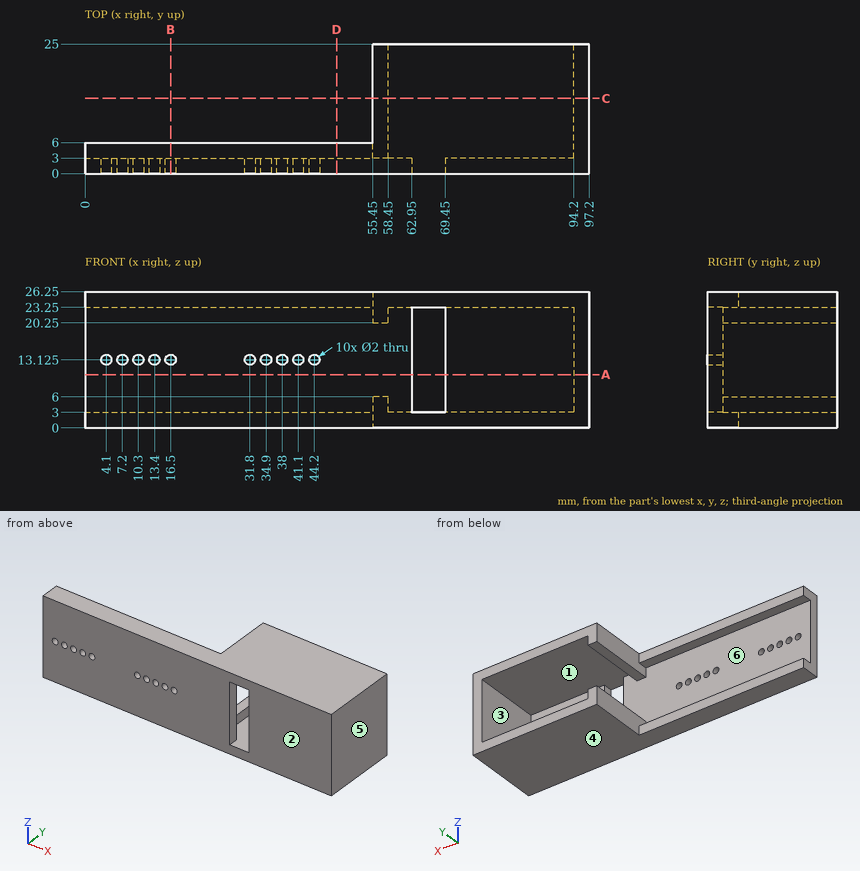
Input: dimensioned drawing with shaded views. Units: mm. Origin: part minimum x, y, z. A direction names the side the tool comes from. Give positions to 0.01 mm unless a question says otherwise; leave off trailing zeros. Order: outer loops, then holes, each group sorted by start corner. A loop starts at its lowest first (then second) coordinate and runs counter-clockwise, first axis right, second up.
(1) Access query for the marked faces 1 and 2. Directions: +Z, -Z, +X, -X, +Y, -Y. A direction counts if a zero-diameter tool reaches every point of the face in a straight line with its end or side. Return the directions, or none.
(2) Contact query for flat-ended pins moving along their axis: P1, Ø1, axis at x = 14, z = 18, coming from the +Y side; P2, Ø3, axis at y = 19.5, z = 22.5, coming from the -X side; P3, Ø0.9, axis at x = 26, z = 24.5, coming from the +Y side. Output: stop coordinate, or through.
(3) Pull-direction query (Z, two-part tool) for the marked faces 3, 4, 5 and 6; classes: +Z half, -Z half, draft (parallel to the pull), parting line (faces both ways), or undercut.
(4) Section query C-C (y = 14.5). Return the cut outline in (x, z).
(5) Section query D-D (x = 48.5). Return the cut outline in (y, z), plus the area to 4 significant figures.
(6) Material intervals for line 1 along Z through (x, y) = (44.2, 2.1) (3 decimals); line 2 along X through (y, z) = (14.75, 21.5); line 3 along Z through (x, y) = (92.5, 21), sorted ascending.
(7) Section query A-A (z = 10.25). Return the cut outline in (x, y), plus the area to 3 significant figures.
(8) Section query B-B (x = 16.5). Return the cut outline in (y, z) (3 decimals).
Outcome:
1. face 1: +Y
1. face 2: +Z, -Z, +X, -X, -Y
2. P1: stops at y = 3
2. P2: stops at x = 55.45
2. P3: stops at y = 6
3. face 3: undercut
3. face 4: -Z half
3. face 5: draft
3. face 6: undercut
4. outline: (55.45, 0) - (97.2, 0) - (97.2, 26.25) - (55.45, 26.25) - (55.45, 20.25) - (58.45, 20.25) - (58.45, 23.25) - (94.2, 23.25) - (94.2, 3) - (58.45, 3) - (58.45, 6) - (55.45, 6) - close
5. outline: (0, 0) - (6, 0) - (6, 3) - (3, 3) - (3, 23.25) - (6, 23.25) - (6, 26.25) - (0, 26.25) - close
5. area: 96.75 mm2
6. line 1: z = 0 to 12.125, 14.125 to 26.25
6. line 2: x = 55.45 to 58.45, 94.2 to 97.2
6. line 3: z = 0 to 3, 23.25 to 26.25
7. outline: (0, 0) - (62.95, 0) - (62.95, 3) - (0, 3) - close; (69.45, 0) - (97.2, 0) - (97.2, 25) - (94.2, 25) - (94.2, 3) - (69.45, 3) - close
7. area: 338 mm2
8. outline: (0, 0) - (6, 0) - (6, 3) - (3, 3) - (3, 12.125) - (0, 12.125) - close; (0, 14.125) - (3, 14.125) - (3, 23.25) - (6, 23.25) - (6, 26.25) - (0, 26.25) - close
